The model under review builds one solid part; all positions refer to its coordinate system, in mm. Face numbers are marked on the shaded views. A direction names the side the tool comes from. Round coordinates to 2 decimals unless told otherwise and drop trailing zeros. Loops run counter-clockwise (first coordinate to the right, second up) from the corner with the lowest first, then second, coordinate; pieces in that order, holes last. Notation, with made-up numbers: M 4,74.5 L 16,74.5 A31 ccw 16,101.5 Z; hole C -7.75,71 d6. An arc over 180 degrees is marked long. Return JSON: item names as keys, results as strings. Group by question number.
Q1. Consider section D-D (z = -59). State the section outline as (x, y) points, and give its area (3 significant figures).
Q2. Draft analysis for pull direction X (two halves, no side actions). For the marked faces 1, 2 and 3, state which applies: pulls with the +X half, pulls with the -X half, needs draft (parallel to the pull), parting line crosses it, or undercut.
Q3. Consider section C-C (y = 59). State the section outline as (x, z) points.
Q4. To check wall thickness, follow line 1 along X through (y, z) = (71, 22); line 2 along X through (y, z) = (19.5, -1); line 3 along Y through (x, z) = (-25, 55). State the ranges of each line that lie inside material, in increasing order.
Q5. Clearance check with flat-ended pins moving along their axes: pin 1 Ø11 at (x, z) = (0, 52) entering from -Y; pin 2 Ø2 at (x, y) = (6, -1) entering from -Z; pin 3 Ø6.5 at (x, y) = (-2.5, -11) entering from +Z; pin 4 Ø14.5 at (y, z) = (-10.5, 19.5) entering from -X. State where each tip first meets the part, or that it passes through.
Q6. Consider section A-A (z = -31.5). State the section outline as (x, y) points.
Q7. Consider section B-B (z = 25). State the section outline as (x, y) points.
Q8. For the marked faces 4, 5, 6, 7 and 8, list the 3-axis set-ups (+Z, -Z, +X, -X, +Y, -Y) from which the entire face can be reached by the end or side of a thin tool; tool diameter is ignored.
from build123d import *

# Parameters (mm, degrees)
SKETCH1_W           = 10
SKETCH1_H           = 80
SKETCH1_W_2         = 3
SKETCH1_W_3         = 80
SKETCH1_H_2         = 3
SKETCH1_H_3         = 10
SKETCH1_W_4         = 30
BOSS_EXTRUDE1_DEPTH = 41.657
SKETCH1_6_W         = 3
SKETCH1_6_H         = 80
SKETCH1_6_W_2       = 80
SKETCH1_6_H_2       = 3
SKETCH1_6_W_3       = 50
BOSS_EXTRUDE2_DEPTH = 70
CUT_EXTRUDE1_REACH  = 170.841
SKETCH2_R           = 3.2639
CUT_EXTRUDE2_REACH  = 145.243
SKETCH3_R           = 3.2639
SKETCH4_W           = 98
SKETCH4_H           = 1.9
BOSS_EXTRUDE3_DEPTH = 5
SKETCH4_4_W         = 98
SKETCH4_4_H         = 1.9
BOSS_EXTRUDE4_DEPTH = 19.05
CUT_EXTRUDE3_DEPTH  = 135.675178822
SKETCH6_R           = 3.2639
BOSS_EXTRUDE5_DEPTH = 5
SKETCH6_3_R         = 3.2639
BOSS_EXTRUDE6_DEPTH = 19.05
SKETCH7_W           = 50
SKETCH7_H           = 25
CUT_EXTRUDE4_DEPTH  = 144.24312825
CHAMFER1_SIZE       = 30
CHAMFER2_SIZE       = 1
CHAMFER2_SIZE2      = 0.577350269
FILLET1_R           = 2


with BuildPart() as part:
    # Sketch1 → Boss-Extrude1 (new body)
    with BuildSketch(Plane.XY):
        with Locations((-49.798838448, 37.726897406)):
            Rectangle(SKETCH1_W, SKETCH1_H)
        with Locations((-56.298838448, 37.726897406)):
            Rectangle(SKETCH1_W_2, SKETCH1_H)
        Polygon((-35.798838448, 87.726897406), (-35.798838448, 84.726897406), (-44.798838448, 77.726897406), (-54.798838448, 77.726897406), (-57.798838448, 77.726897406), (-35.798838448, 90.726897406), align=None)
        with Locations((4.201161552, 86.226897406)):
            Rectangle(SKETCH1_W_3, SKETCH1_H_2)
        with Locations((4.201161552, 89.226897406)):
            Rectangle(SKETCH1_W_3, SKETCH1_H_2)
        Polygon((44.201161552, 87.726897406), (44.201161552, 90.726897406), (66.201161552, 77.726897406), (63.201161552, 77.726897406), (53.201161552, 77.726897406), (44.201161552, 84.726897406), align=None)
        with Locations((58.201161552, 37.726897406)):
            Rectangle(SKETCH1_W, SKETCH1_H)
        with Locations((64.701161552, 37.726897406)):
            Rectangle(SKETCH1_W_2, SKETCH1_H)
        with Locations((4.201161552, -7.273102594)):
            Rectangle(SKETCH1_W_3, SKETCH1_H_3)
        Polygon((66.201161552, -2.273102594), (44.201161552, -15.273102594), (44.201161552, -12.273102594), (44.201161552, -2.273102594), (53.201161552, -2.273102594), (63.201161552, -2.273102594), align=None)
        Polygon((-35.798838448, -15.273102594), (-57.798838448, -2.273102594), (-54.798838448, -2.273102594), (-44.798838448, -2.273102594), (-35.798838448, -2.273102594), (-35.798838448, -12.273102594), align=None)
        with Locations((4.201161552, -13.773102594)):
            Rectangle(SKETCH1_W_3, SKETCH1_H_2)
        with Locations((29.201161552, -13.773102594)):
            Rectangle(SKETCH1_W_4, SKETCH1_H_2)
    extrude(amount=BOSS_EXTRUDE1_DEPTH)

    # Sketch1<6> → Boss-Extrude2 (add)
    with BuildSketch(Plane.XY):
        with Locations((-56.298838448, 37.726897406)):
            Rectangle(SKETCH1_6_W, SKETCH1_6_H)
        with Locations((4.201161552, 89.226897406)):
            Rectangle(SKETCH1_6_W_2, SKETCH1_6_H_2)
        with Locations((-10.798838448, -13.773102594)):
            Rectangle(SKETCH1_6_W_3, SKETCH1_6_H_2)
        with Locations((64.701161552, 37.726897406)):
            Rectangle(SKETCH1_6_W, SKETCH1_6_H)
    extrude(amount=-BOSS_EXTRUDE2_DEPTH)

    # Sketch2 → Cut-Extrude1 (cut, up to next)
    with BuildSketch(Plane.ZY.offset(57.798838448), mode=Mode.PRIVATE) as cut_extrude1_sk1:
        with Locations(Location((-59, 37.726897406, 0), (0, 0, 270))):
            Circle(SKETCH2_R)
    cut_extrude1_tool1 = extrude(cut_extrude1_sk1.sketch, amount=-CUT_EXTRUDE1_REACH, mode=Mode.PRIVATE) & part.part
    add(cut_extrude1_tool1.solids().sort_by_distance((-57.798838, 37.726897, -59))[0], mode=Mode.SUBTRACT)

    # Sketch3 → Cut-Extrude2 (cut, up to next)
    with BuildSketch(Plane(origin=(0, 90.726897406, 0), x_dir=(1, 0, 0), z_dir=(0, 1, 0)), mode=Mode.PRIVATE) as cut_extrude2_sk1:
        with Locations(Location((4.201161552, 59, 0), (0, 0, 270))):
            Circle(SKETCH3_R)
    cut_extrude2_tool1 = extrude(cut_extrude2_sk1.sketch, amount=-CUT_EXTRUDE2_REACH, mode=Mode.PRIVATE) & part.part
    add(cut_extrude2_tool1.solids().sort_by_distance((4.201162, 90.726897, -59))[0], mode=Mode.SUBTRACT)

    # Sketch4 → Boss-Extrude3 (add)
    with BuildSketch(Plane.XY.offset(41.657)):
        Polygon((51.786875838, 78.826897406), (64.33962309, 78.826897406), (44.201161552, 90.726897406), (-35.798838448, 90.726897406), (-55.937299987, 78.826897406), (-43.384552734, 78.826897406), (-35.798838448, 84.726897406), (44.201161552, 84.726897406), align=None)
        Polygon((-43.384552734, 78.826897406), (51.786875838, 78.826897406), (44.201161552, 84.726897406), (-35.798838448, 84.726897406), align=None)
        Polygon((53.201161552, 75.826897406), (66.201161552, 75.826897406), (66.201161552, 77.726897406), (64.33962309, 78.826897406), (51.786875838, 78.826897406), (53.201161552, 77.726897406), align=None)
        Polygon((-44.798838448, 75.826897406), (53.201161552, 75.826897406), (53.201161552, 77.726897406), (51.786875838, 78.826897406), (-43.384552734, 78.826897406), (-44.798838448, 77.726897406), align=None)
        Polygon((66.201161552, -2.273102594), (66.201161552, -0.373102594), (53.201161552, -0.373102594), (53.201161552, -2.273102594), (-44.798838448, -2.273102594), (-44.798838448, -0.373102594), (-57.798838448, -0.373102594), (-57.798838448, -2.273102594), (-55.937299987, -3.373102594), (64.33962309, -3.373102594), align=None)
        with Locations((4.201161552, -1.323102594)):
            Rectangle(SKETCH4_W, SKETCH4_H)
        Polygon((44.201161552, -15.273102594), (64.33962309, -3.373102594), (-55.937299987, -3.373102594), (-35.798838448, -15.273102594), align=None)
        Polygon((-57.798838448, 75.826897406), (-44.798838448, 75.826897406), (-44.798838448, 77.726897406), (-43.384552734, 78.826897406), (-55.937299987, 78.826897406), (-57.798838448, 77.726897406), align=None)
    extrude(amount=BOSS_EXTRUDE3_DEPTH)

    # Sketch4<4> → Boss-Extrude4 (add)
    with BuildSketch(Plane.XY.offset(41.657)):
        Polygon((53.201161552, 75.826897406), (66.201161552, 75.826897406), (66.201161552, 77.726897406), (64.33962309, 78.826897406), (51.786875838, 78.826897406), (53.201161552, 77.726897406), align=None)
        Polygon((-44.798838448, 75.826897406), (53.201161552, 75.826897406), (53.201161552, 77.726897406), (51.786875838, 78.826897406), (-43.384552734, 78.826897406), (-44.798838448, 77.726897406), align=None)
        Polygon((66.201161552, -2.273102594), (66.201161552, -0.373102594), (53.201161552, -0.373102594), (53.201161552, -2.273102594), (-44.798838448, -2.273102594), (-44.798838448, -0.373102594), (-57.798838448, -0.373102594), (-57.798838448, -2.273102594), (-55.937299987, -3.373102594), (64.33962309, -3.373102594), align=None)
        with Locations((4.201161552, -1.323102594)):
            Rectangle(SKETCH4_4_W, SKETCH4_4_H)
        Polygon((-57.798838448, 75.826897406), (-44.798838448, 75.826897406), (-44.798838448, 77.726897406), (-43.384552734, 78.826897406), (-55.937299987, 78.826897406), (-57.798838448, 77.726897406), align=None)
    extrude(amount=BOSS_EXTRUDE4_DEPTH)

    # Sketch5 → Cut-Extrude3 (cut, through all)
    with BuildSketch(Plane.XZ.offset(3.373102594)):
        with BuildLine():
            Line((-49.862738448, 60.707), (-49.862738448, 54.357))
            ThreePointArc((-49.862738448, 54.357), (-46.598838448, 51.0931), (-43.334938448, 54.357))
            Line((-43.334938448, 54.357), (-43.334938448, 60.707))
            Line((-43.334938448, 60.707), (-49.862738448, 60.707))
        make_face()
        with BuildLine():
            Line((51.737261552, 60.707), (51.737261552, 54.357))
            ThreePointArc((51.737261552, 54.357), (55.001161552, 51.0931), (58.265061552, 54.357))
            Line((58.265061552, 54.357), (58.265061552, 60.707))
            Line((58.265061552, 60.707), (51.737261552, 60.707))
        make_face()
    extrude(amount=-CUT_EXTRUDE3_DEPTH, mode=Mode.SUBTRACT)

    # Sketch6 → Boss-Extrude5 (add)
    # profile 1 of 2: a face of its own
    with BuildSketch(Plane.XY.offset(41.657)):
        with BuildLine():
            Line((-44.798838448, 42.726897406), (-44.798838448, 37.726897406))
            Line((-44.798838448, 37.726897406), (-44.798838448, 32.726897406))
            Line((-44.798838448, 32.726897406), (-21.198838448, 32.726897406))
            ThreePointArc((-21.198838448, 32.726897406), (-16.198838448, 37.726897406), (-21.198838448, 42.726897406))
            Line((-21.198838448, 42.726897406), (-44.798838448, 42.726897406))
        make_face()
        with Locations((-21.198838448, 37.726897406)):
            Circle(SKETCH6_R, mode=Mode.SUBTRACT)
    # profile 2 of 2: a face of its own
    with BuildSketch(Plane.XY.offset(41.657)):
        with Locations((-21.198838448, 37.726897406)):
            Circle(SKETCH6_R)
    extrude(amount=-BOSS_EXTRUDE5_DEPTH)

    # Sketch6<3> → Boss-Extrude6 (add)
    with BuildSketch(Plane.XY.offset(41.657)):
        with Locations(Location((-21.198838448, 37.726897406, 0), (0, 0, 180))):
            Circle(SKETCH6_3_R)
    extrude(amount=BOSS_EXTRUDE6_DEPTH)

    # Sketch7 → Cut-Extrude4 (cut, through all)
    with BuildSketch(Plane(origin=(0, 90.726897406, 0), x_dir=(1, 0, 0), z_dir=(0, 1, 0))):
        with Locations((4.201161552, -20.5)):
            Rectangle(SKETCH7_W, SKETCH7_H)
    extrude(amount=-CUT_EXTRUDE4_DEPTH, mode=Mode.SUBTRACT)

    # Chamfer1
    # the kernel refuses this chamfer: 30 mm, written as the material it takes off along each edge
    with BuildSketch(Plane(origin=(22.351651191, 77.726897406, -70), x_dir=(0, 0.02749587661058632, 0.9996219169112968), z_dir=(-1, 0, 0)), Plane(origin=(-134.949328087, -2.273102594, -70), x_dir=(0, -0.02749587661058638, 0.9996219169112968), z_dir=(1, 0, 0)), Plane(origin=(-35.798838448, 64.877387045, -70), x_dir=(-0.02749587661058632, 0, 0.9996219169112968), z_dir=(0, -1, 0)), Plane(origin=(14.201161552, -92.423592233, -70), x_dir=(0.02749587661058638, 0, 0.9996219169112968), z_dir=(0, 1, 0)), Plane(origin=(-13.949328087, -2.273102594, -70), x_dir=(0, -0.02749587661058636, 0.9996219169112968), z_dir=(1, 0, 0)), Plane(origin=(143.351651191, 77.726897406, -70), x_dir=(0, 0.02749587661058632, 0.9996219169112968), z_dir=(-1, 0, 0)), Plane(origin=(44.201161552, 10.576407767, -70), x_dir=(0.02749587661058632, 0, 0.9996219169112968), z_dir=(0, 1, 0)), Plane(origin=(-35.798838448, 167.877387045, -70), x_dir=(-0.02749587661058632, 0, 0.9996219169112968), z_dir=(0, -1, 0))) as chamfer1_piece_1:
        Polygon((CHAMFER1_SIZE * 0.999621916911, -CHAMFER1_SIZE * 0.0274958766106), (-CHAMFER1_SIZE * 0.0274958766106, -CHAMFER1_SIZE * 0.999621916911), (0, 0), align=None)
    extrude(amount=157.300979278, mode=Mode.SUBTRACT)

    # Chamfer2
    chamfer2_edges = [part.edges().sort_by_distance(p)[0] for p in [
        (-17.934938448, 37.726897406, 60.707),
    ]]
    chamfer2_side = [part.faces().sort_by_distance(p)[0] for p in [
        (-17.934938448, 37.726897406, 51.182),
    ]]
    chamfer(chamfer2_edges, length=CHAMFER2_SIZE, length2=CHAMFER2_SIZE2, reference=chamfer2_side[0])

    # Fillet1
    fillet1_edges = [part.edges().sort_by_distance(p)[0] for p in [
        (66.201161552, -1.323102594, 60.707),
        (-57.798838448, -1.323102594, 60.707),
        (-57.798838448, 76.776897406, 60.707),
        (66.201161552, 76.776897406, 60.707),
        (58.265061552, 77.326897406, 60.707),
        (51.737261552, 77.326897406, 60.707),
        (-43.334938448, 77.326897406, 60.707),
        (-49.862738448, 77.326897406, 60.707),
        (-49.862738448, -1.873102594, 60.707),
        (-43.334938448, -1.873102594, 60.707),
        (51.737261552, -1.873102594, 60.707),
        (58.265061552, -1.873102594, 60.707),
        (-44.798838448, 32.726897406, 39.157),
        (-44.798838448, 42.726897406, 39.157),
        (14.201161552, 89.226897406, -70),
        (-5.798838448, 89.226897406, -70),
        (-35.798838448, 89.226897406, -40),
        (-56.298838448, 77.726897406, -40),
        (-56.298838448, 27.726897406, -70),
        (-56.298838448, 47.726897406, -70),
        (-56.298838448, -2.273102594, -40),
        (-35.798838448, -13.773102594, -40),
        (14.201161552, -13.773102594, -40),
        (64.701161552, -2.273102594, -40),
        (64.701161552, 47.726897406, -70),
        (64.701161552, 27.726897406, -70),
        (64.701161552, 77.726897406, -40),
        (44.201161552, 89.226897406, -40),
        (-10.798838448, -13.773102594, -65),
    ]]
    fillet(fillet1_edges, radius=FILLET1_R)


solid = part.part
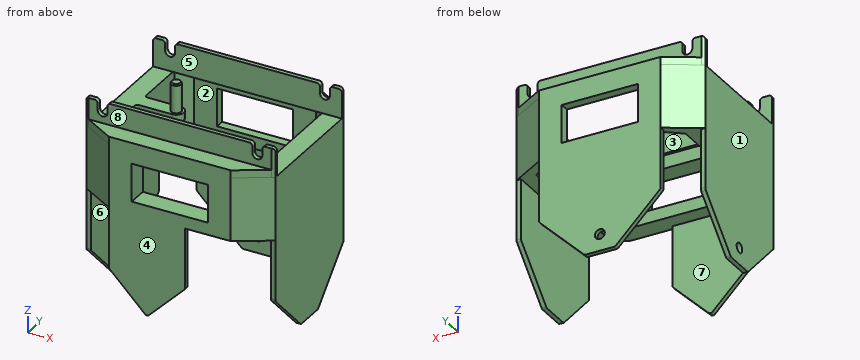
Values:
{
 "1": {"outline": "M -57.8,16.73 L -54.8,16.73 L -54.8,34.46 L -57.8,34.46 Z; M -57.8,40.99 L -54.8,40.99 L -54.8,58.73 L -57.8,58.73 Z; M -16.8,-15.27 L -4.8,-15.27 L -4.8,-12.27 L -16.8,-12.27 Z; M -16.8,87.73 L 0.94,87.73 L 0.94,90.73 L -16.8,90.73 Z; M 7.47,87.73 L 25.2,87.73 L 25.2,90.73 L 7.47,90.73 Z; M 63.2,16.73 L 66.2,16.73 L 66.2,58.73 L 63.2,58.73 Z", "area": "375 mm2"},
 "2": {"face 1": "pulls with the -X half", "face 2": "undercut", "face 3": "needs draft"},
 "3": {"outline": "M -57.8,-58.73 L -54.8,-58.73 L -54.8,0 L -44.8,0 L -44.8,41.66 L -57.8,41.66 Z; M 53.2,0 L 63.2,0 L 63.2,-58.73 L 66.2,-58.73 L 66.2,41.66 L 53.2,41.66 Z"},
 "4": {"line 1": "x = -57.8 to -44.8, 53.2 to 66.2", "line 2": "x = -57.8 to -54.8, 63.2 to 66.2", "line 3": "y = -3.37 to -0.37, 75.83 to 78.83"},
 "5": {"pin 1": "stops at y = -15.27", "pin 2": "stops at z = 41.66", "pin 3": "stops at z = 46.66", "pin 4": "stops at x = -56.15"},
 "6": {"outline": "M -57.8,-2.27 L -54.8,-2.27 L -54.8,77.73 L -57.8,77.73 Z; M -35.8,-15.27 L 14.2,-15.27 L 14.2,-12.27 L -35.8,-12.27 Z; M -35.8,87.73 L 44.2,87.73 L 44.2,90.73 L -35.8,90.73 Z; M 63.2,-2.27 L 66.2,-2.27 L 66.2,77.73 L 63.2,77.73 Z"},
 "7": {"outline": "M -57.8,-2.27 L -35.8,-15.27 L -20.8,-15.27 L -20.8,-2.27 L -44.8,-2.27 L -44.8,77.73 L -35.8,84.73 L -20.8,84.73 L -20.8,90.73 L -35.8,90.73 L -57.8,77.73 Z; M 29.2,-15.27 L 44.2,-15.27 L 66.2,-2.27 L 66.2,77.73 L 44.2,90.73 L 29.2,90.73 L 29.2,84.73 L 44.2,84.73 L 53.2,77.73 L 53.2,-2.27 L 29.2,-2.27 Z"},
 "8": {"face 4": "+Z, -Z, +X, -X, -Y", "face 5": "+Z, +X, -X", "face 6": "-Z, +Y, -Y", "face 7": "-Z, +X, -X", "face 8": "+Z, +X, -X, -Y"}
}
